The model under review builds one solid part; all positions refer to its coordinate system, in mm. Face numbers are marked on the shaded views. A direction names the side the tool comes from. Coordinates: 2 decimals unless noted, no trailing zeros. Loops run counter-clockwise (first coordinate to the right, second up) from the corner with the lowest first, then second, coordinate; pieces in that order, holes last. Notation, with made-up numbers: M -35,53 L 9,53 A29 cw 9,86 Z; hole C 32,-10 d1. An arc over 180 degrees is marked long. Use one line per item in the form item = value.
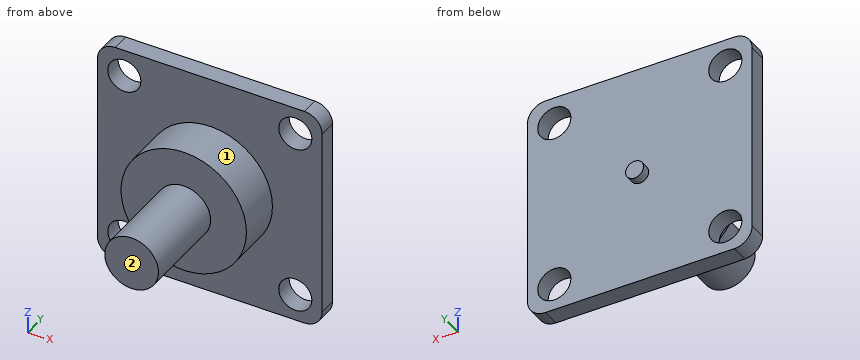
Autodesk Inventor part; units mm, degrees
ref_plane "YZ Plane" through (0, 0, 0) normal (1, 0, 0) x (0, 1, 0)
ref_plane "XZ Plane" through (0, 0, 0) normal (0, 1, 0) x (-1, 0, 0)
ref_plane "XY Plane" through (0, 0, 0) normal (0, 0, 1) x (1, 0, 0)
sketch "Sketch1" plane through (0, 0, 0) normal (0, 1, 0) x (-1, 0, 0)
  line L0 (12.55, 12.55) -> (-12.55, 12.55)
  line L1 (-12.55, 12.55) -> (-12.55, -12.55)
  line L2 (-12.55, -12.55) -> (12.55, -12.55)
  line L3 (12.55, -12.55) -> (12.55, 12.55)
  point P0 (0, 0)
  point P1 (12.55, 0)
  point P2 (0, -12.55)
  dimension "d0" = 25.1
  dimension "d1" = 25.1
extrude "Extrusion1" add sketch "Sketch1" along normal blind 2
fillet "Fillet1" radius 2 4 edges at (12.55, 1, 12.55) (-12.55, 1, 12.55) (12.55, 1, -12.55) (-12.55, 1, -12.55)
sketch "Sketch2" plane through (0, 2, 0) normal (0, 1, 0) x (1, 0, 0)
  circle A0 centre (-9.55, -9.55) radius 1.85
  line L0 (-12.55, 10.55) -> (-12.55, -10.55)
  line L1 (-10.55, -12.55) -> (10.55, -12.55)
  line L2 (0, 0) -> (-4.3818, 0) construction
  line L3 (0, 0) -> (0, 4.1079) construction
  circle A1 centre (-9.55, 9.55) radius 1.85
  circle A2 centre (9.55, -9.55) radius 1.85
  circle A3 centre (9.55, 9.55) radius 1.85
  dimension "d5" = 3.7
  dimension "d6" = 3
  dimension "d7" = 3
extrude "Extrusion2" cut sketch "Sketch2" against normal through all
sketch "Sketch3" plane through (0, 2, 0) normal (0, 1, 0) x (1, 0, 0)
  circle A0 centre (0, 0) radius 1
  dimension "d10" = 2
extrude "Extrusion3" add sketch "Sketch3" along normal blind 1
sketch "Sketch4" plane through (0, 0, 0) normal (0, -1, 0) x (1, 0, 0)
  circle A0 centre (0, 0) radius 1
  circle A1 centre (0, 0) radius 7
  dimension "d13" = 14
extrude "Extrusion4" add sketch "Sketch4" along normal blind 5 contours A0 | A1
sketch "Sketch5" plane through (0, -5, 0) normal (0, -1, 0) x (1, 0, 0)
  circle A0 centre (0, 0) radius 1
  circle A1 centre (0, 0) radius 3
  dimension "d16" = 6
extrude "Extrusion5" add sketch "Sketch5" along normal blind 10 contours A0 | A1
properties part number "connector" material "Aluminum 6061"
1. Add section A-A (x = 9.55). State the section outline as (y, z) points.
Response values:
outline = M 0,-12.55 L 2,-12.55 L 2,-11.4 L 0,-11.4 Z; M 0,-7.7 L 2,-7.7 L 2,7.7 L 0,7.7 Z; M 0,11.4 L 2,11.4 L 2,12.55 L 0,12.55 Z
2. Insertion check: P1, Ø2, axis at x = 3.5, z = -1.5, coming from the +Y side; P2, Ø8, axis at y = -7.5, z = -5, coming from the +X side; P3, Ø3, axis at x = 9.55, z = -9.55, coming from the -Y side; P4, Ø10, axis at y = -10, z = 7.5, coming from the +X side. Each pin has a flat end and moves straight along its axis. Give the tip position at first contact, or say it passes through.
Response values:
P1 = 2
P2 = 6.74
P3 = through
P4 = 1.66
3. Add section B-B (z = -9.55). State the section outline as (x, y) points.
Response values:
outline = M -12.55,0 L -11.4,0 L -11.4,2 L -12.55,2 Z; M -7.7,0 L 7.7,0 L 7.7,2 L -7.7,2 Z; M 11.4,0 L 12.55,0 L 12.55,2 L 11.4,2 Z
4. Machinability: for the marked faces 1 and 2, which of the approach directions +Z, -Z, +X, -X, +Y, -Y give a long, thin tool a straight path to every point of the face, cutting with its end or side? Answer none if there is none.
Response values:
face_1 = -Y
face_2 = +Z, -Z, +X, -X, -Y
5. Add section C-C (y = 1). State the section outline as (x, z) points, then the cut area to 3 significant figures.
Response values:
outline = M -12.55,-10.55 A2 ccw -10.55,-12.55 L 10.55,-12.55 A2 ccw 12.55,-10.55 L 12.55,10.55 A2 ccw 10.55,12.55 L -10.55,12.55 A2 ccw -12.55,10.55 Z; hole C -9.55,-9.55 d3.7; hole C -9.55,9.55 d3.7; hole C 9.55,-9.55 d3.7; hole C 9.55,9.55 d3.7
area = 584 mm^2
6. Add section D-D (x = 0). State the section outline as (y, z) points, then the cut area to 3 significant figures.
Response values:
outline = M -15,-3 L -5,-3 L -5,-7 L 0,-7 L 0,-12.55 L 2,-12.55 L 2,-1 L 3,-1 L 3,1 L 2,1 L 2,12.55 L 0,12.55 L 0,7 L -5,7 L -5,3 L -15,3 Z
area = 182 mm^2
7. Wall thickness on line 1 along X through (y, z) = (1.3, 9.55); line 2 along X through (y, z) = (1.5, 10): over which ranges is each line inside the solid? List them lowest first. Write a range as from..to.
Response values:
line_1 = -12.55..-11.4, -7.7..7.7, 11.4..12.55
line_2 = -12.55..-11.34, -7.76..7.76, 11.34..12.55
